Could you check a few things on this model? Use its own coordinates, in mm. A direction names the side the tool comes from. Give positions to 0.01 mm unless a question says otherwise; leave off trailing zeros. Loops run counter-clockwise (first coordinate to the right, second up) from the corner with the lowest first, then second, coordinate; pieces in that order, holes last. Notation, with made-up numbers: M 80.25,-40 L 89.25,-40 A26 ccw 89.25,-8 Z; hole C -2,35 d11. An arc over 180 degrees is marked long. Use a Markdown table: item, result. Add a question column.
1) Which directions (+Z, -Z, +X, -X, +Y, -Y) give clear straight access to the entire face, cutting with the end or side of a thin tool? Please do faces 4 (the flat face through (-3, 12.299, 2)), 5 (the flat face through (-2, -16, -2)).
2) Suppose I cut it at A-A on z = 4. List the corners of the cut face in (x, y) for me.
3) Suppose I cut it at B-B on y = -9.5. List the corners of the cut face in (x, z) for me.
4) If I drill on line 1 along X through (y, z) = (-37.5, 3.25); line 2 along Y through (x, z) = (-18, 1); line 3 along Z through (x, y) = (-0.5, 9.5), over which ranges is the centre line in solid material (lowest first)? Write a range as [from, to].
5) Suppose I cut it at C-C on x = 23. List the corners of the cut face in (y, z) for me.
6) We'd pull the mould along Y, two halves only. Please class faces 1 (the flat face through (-2, 14.299, 2)), 2 (the flat face through (42.237, -17, 2)), 3 (the flat face through (-2, -16, 0)): +Y half, -Y half, draft (parallel to the pull), parting line (faces both ways), or undercut.
7) Will this pin go through, and if not, where does the flat tip stop? pin 1 Ø17 at (x, y) = (0.5, -4.5) entering from +Z.
```python
from build123d import *

# Parameters (mm, degrees)
ESBO_O1_W                = 89
ESBO_O1_H                = 61
ESBO_O1_W_2              = 85
ESBO_O1_H_2              = 57
RESSALTO_EXTRUS_O1_DEPTH = 5
ESBO_O2_W                = 89
ESBO_O2_H                = 61
RESSALTO_EXTRUS_O2_DEPTH = 2
FILETE6_R                = 1
FILETE7_R                = 1
FILETE10_R               = 1
FILETE11_R               = 1
FILETE12_R               = 1


with BuildPart() as part:
    # Esboço1 → Ressalto-extrusão1 (new body)
    with BuildSketch(Plane.XY):
        with Locations((-2.263340114, -16.201421801)):
            Rectangle(ESBO_O1_W, ESBO_O1_H)
        with Locations((-2.263340114, -16.201421801)):
            Rectangle(ESBO_O1_W_2, ESBO_O1_H_2, mode=Mode.SUBTRACT)
    extrude(amount=RESSALTO_EXTRUS_O1_DEPTH)

    # Esboço2 → Ressalto-extrusão2 (add)
    with BuildSketch(Plane(origin=(0, 0, 0), x_dir=(-1, 0, 0), z_dir=(0, 0, -1))):
        with Locations((2.263340114, -16.201421801)):
            Rectangle(ESBO_O2_W, ESBO_O2_H)
    extrude(amount=RESSALTO_EXTRUS_O2_DEPTH)

    # Filete6
    filete6_edges = [part.edges().sort_by_distance(p)[0] for p in [
        (40.236659886, 12.298578199, 2.5),
    ]]
    fillet(filete6_edges, radius=FILETE6_R)

    # Filete7
    filete7_edges = [part.edges().sort_by_distance(p)[0] for p in [
        (-44.763340114, 12.298578199, 2.5),
        (-44.763340114, -44.701421801, 2.5),
        (40.236659886, -44.701421801, 2.5),
    ]]
    fillet(filete7_edges, radius=FILETE7_R)

    # Filete10
    filete10_edges = [part.edges().sort_by_distance(p)[0] for p in [
        (-46.763340114, -46.701421801, 1.5),
    ]]
    fillet(filete10_edges, radius=FILETE10_R)

    # Filete11
    filete11_edges = [part.edges().sort_by_distance(p)[0] for p in [
        (-46.763340114, 14.298578199, 1.5),
        (42.236659886, 14.298578199, 1.5),
        (42.236659886, -46.701421801, 1.5),
    ]]
    fillet(filete11_edges, radius=FILETE11_R)

    # Filete12
    filete12_edges = [part.edges().sort_by_distance(p)[0] for p in [
        (-46.763340114, -16.201421801, -2),
        (-46.470446895, -46.408528582, -2),
        (42.236659886, -16.201421801, -2),
        (-2.263340114, -46.701421801, -2),
        (-2.263340114, 14.298578199, -2),
        (-46.470446895, 14.00568498, -2),
        (41.943766667, 14.00568498, -2),
        (41.943766667, -46.408528582, -2),
    ]]
    fillet(filete12_edges, radius=FILETE12_R)


solid = part.part
```
Answer block:
| question | item | result |
|---|---|---|
| 1 | face 4 | +Z |
| 1 | face 5 | -Z, +X, -X, +Y, -Y |
| 2 | outline | M -46.76,-45.7 A1 ccw -45.76,-46.7 L 41.24,-46.7 A1 ccw 42.24,-45.7 L 42.24,13.3 A1 ccw 41.24,14.3 L -45.76,14.3 A1 ccw -46.76,13.3 Z; hole M -44.76,-43.7 A1 ccw -43.76,-44.7 L 39.24,-44.7 A1 ccw 40.24,-43.7 L 40.24,11.3 A1 ccw 39.24,12.3 L -43.76,12.3 A1 ccw -44.76,11.3 Z |
| 3 | outline | M -46.76,-1 A1 ccw -45.76,-2 L 41.24,-2 A1 ccw 42.24,-1 L 42.24,5 L 40.24,5 L 40.24,0 L -44.76,0 L -44.76,5 L -46.76,5 Z |
| 4 | line 1 | x = [-46.76, -44.76], [40.24, 42.24] |
| 4 | line 2 | y = [-46.7, -44.7], [12.3, 14.3] |
| 4 | line 3 | z = [-2, 0] |
| 5 | outline | M -46.7,-1 A1 ccw -45.7,-2 L 13.3,-2 A1 ccw 14.3,-1 L 14.3,5 L 12.3,5 L 12.3,0 L -44.7,0 L -44.7,5 L -46.7,5 Z |
| 6 | face 1 | +Y half |
| 6 | face 2 | draft |
| 6 | face 3 | undercut |
| 7 | pin 1 | stops at z = 0 |
